Check sheet for the modelled part. Datum: model origin and axes. Units: mm. A direction names the side the tool comes from. Coordinates: 2 decimals unless noted, no trailing zeros. Order: outer loops, then holes, each group sorted by start corner. A loop starts at its lowest first (then second) coordinate and runs counter-clockwise, first axis right, second up. Notation, with made-up numbers: M 48.5,50.25 L 75.5,50.25 A26 ccw 75.5,71.25 Z; hole C 51.5,-11 d2. An arc over 180 degrees is marked long. Answer in a Markdown table with one row per item. Add a question column.
Autodesk Inventor part; units mm, degrees
ref_plane "YZ Plane" through (0, 0, 0) normal (1, 0, 0) x (0, 1, 0)
ref_plane "XZ Plane" through (0, 0, 0) normal (0, 1, 0) x (-1, 0, 0)
ref_plane "XY Plane" through (0, 0, 0) normal (0, 0, 1) x (1, 0, 0)
sketch "スケッチ4" plane through (0, 0, 0) normal (0, 0, 1) x (1, 0, 0)
  circle A0 centre (0, 0) radius 20
  dimension "d22" = 40
extrude "押し出し3" add sketch "スケッチ4" along normal blind 2
sketch "スケッチ5" plane through (0, 0, 2) normal (0, 0, 1) x (1, 0, 0)
  circle A0 centre (0, 0) radius 5
  dimension "d25" = 10
extrude "押し出し4" add sketch "スケッチ5" along normal blind 5
sketch "スケッチ6" plane through (0, 0, 0) normal (0, 0, -1) x (-1, 0, 0)
  circle A0 centre (0, 0) radius 4
  dimension "d28" = 8
extrude "押し出し5" add sketch "スケッチ6" along normal blind 0.5
sketch "スケッチ7" plane through (0, 0, 7) normal (0, 0, 1) x (1, 0, 0)
  circle A0 centre (0, 0) radius 1.5
  dimension "d31" = 3
extrude "押し出し6" cut sketch "スケッチ7" against normal blind 10
properties part number "Gear4_S50B 80B+0203" material "真鍮"
1. Go/stop test with flat-tipped pins: pin 1 Ø4 at (x, y) = (1, 15) entering from +Z; pin 2 Ø20 at (x, y) = (0, -7.5) entering from +Z; pin 3 Ø3 at (y, z) = (-1.5, 5.5) entering from +X; pin 4 Ø3 at (x, y) = (2, 15) entering from -Z. Record where each tip stops, or that it passes through.
2. Section check A-A on y = 0. Enter the section's corners in (x, z).
3. Scan lines: line 1 (Y direction, x = 0, z = 2.75); line 2 (Z direction, x = 6.5, y = 4.5); line 3 (X direction, y = -1, z = 0.75). Record each from-to range of solid material in increasing order.
4. Set-up check for faces 1 (the cylindrical face through (0.867, 3.905, -0.246)), 2 (the flat face through (-2, 0, -0.5)), 3 (the flat face through (4, -4, 2)): record each of +Z, -Z, +X, -X, +Y, -Y from which the full face is reachable in a straight line by a thin tool's end or side.
5. Section check C-C on z = 3.5. Enter the section's corners in (x, y), then the cut area to 3 significant figures.
6. Release check for a two-part mould opening along Y. For faces 4 (the flat face through (4.2, 0.3, 0)), 5 (the cylindrical face through (-1.5, 0.07, 3.3)), 6 (the cylindrical face through (-4.336, 19.524, 0.986)) record: released by +Y, released by -Y, zero draft, split by the parting line, or undercut.
7. Section check D-D on x = -16. Enter the section's corners in (y, z), then the cut area to 3 significant figures.
Result sheet:
| question | item | result |
|---|---|---|
| 1 | pin 1 | z = 2 |
| 1 | pin 2 | z = 7 |
| 1 | pin 3 | x = 5 |
| 1 | pin 4 | z = 0 |
| 2 | outline | M -20,0 L -4,0 L -4,-0.5 L -1.5,-0.5 L -1.5,7 L -5,7 L -5,2 L -20,2 Z; M 1.5,-0.5 L 4,-0.5 L 4,0 L 20,0 L 20,2 L 5,2 L 5,7 L 1.5,7 Z |
| 3 | line 1 | -5 to -1.5, 1.5 to 5 |
| 3 | line 2 | 0 to 2 |
| 3 | line 3 | -19.97 to -1.12, 1.12 to 19.97 |
| 4 | face 1 | -Z |
| 4 | face 2 | -Z, +X, -X, +Y, -Y |
| 4 | face 3 | +Z |
| 5 | outline | C 0,0 d10; hole C 0,0 d3 |
| 5 | area | 71.5 mm^2 |
| 6 | face 4 | zero draft |
| 6 | face 5 | undercut |
| 6 | face 6 | split by the parting line |
| 7 | outline | M -12,0 L 12,0 L 12,2 L -12,2 Z |
| 7 | area | 48.0 mm^2 |
